Check sheet for the modelled part. Datum: model origin and axes. Units: mm. A direction names the side the tool comes from. Round coordinates to 2 decimals unless told otherwise and drop trailing zeros. Write each loop counter-clockwise with the first axis right and the second up, starting at its lowest first coordinate (ties: lowest second). Pieces come first, ordered by that corner, then holes. Notation, with made-up numbers: (-4, -32.5) -> (53, -32.5) arc R38 ccw to (53, 5.5) -> close; hole circle Ø7 at (-14, 20.25). An arc over 180 degrees is marked (long way). One line per item, written item: value.
from build123d import *

# Parameters (mm, degrees)
TORUS_R                = 1
CYLINDER_R             = 5.5
CYLINDER_DEPTH         = 36
FILLET_R               = 4
CYLINDER002_W          = 7
CYLINDER002_H          = 6
CYLINDER002_ANGLE      = 250
FILLET001_R            = 0.5
CUT001_PLACEMENT_ANGLE = 55
BOX_W                  = 8
BOX_H                  = 6
BOX_DEPTH              = 6
BOX001_W               = 2
BOX001_H               = 50
BOX001_DEPTH           = 10


with BuildPart() as toro:
    # Torus → Torus (revolve)
    with BuildSketch(Plane(origin=(0, 0, 26), x_dir=(1, 0, 0), z_dir=(0, -1, 0))):
        with Locations((6, 0)):
            Circle(TORUS_R)
    revolve(axis=Axis((0, 0, 26), (0, 0, 1)))


with BuildPart() as led:
    # Cylinder → Cylinder (new body)
    with BuildSketch(Plane.XY):
        Circle(CYLINDER_R)
    extrude(amount=CYLINDER_DEPTH)

    # Fillet
    fillet_edges = [led.edges().sort_by_distance(p)[0] for p in [
        (-5.5, 0, 36),
    ]]
    fillet(fillet_edges, radius=FILLET_R)

    # Cut: cut Toro
    add(toro.part, mode=Mode.SUBTRACT)


with BuildPart() as obj1:
    # Cylinder002 → Cylinder002 (revolve)
    with BuildSketch(Plane(origin=(0, 0, 4), x_dir=(1, 0, 0), z_dir=(0, -1, 0))):
        with Locations((3.5, 3)):
            Rectangle(CYLINDER002_W, CYLINDER002_H)
    revolve(axis=Axis((0, 0, 4), (0, 0, 1)), revolution_arc=CYLINDER002_ANGLE)

    # Fillet001
    fillet001_edges = [obj1.edges().sort_by_distance(p)[0] for p in [
        (-2.394141, -6.577848, 7),
        (7, 0, 7),
    ]]
    fillet(fillet001_edges, radius=FILLET001_R)


with BuildPart() as obj1_1:
    # Fillet001 placement: moved
    add(obj1.part.moved(Location((0, 0, 19))))

    # Cut001: cut led
    add(led.part, mode=Mode.SUBTRACT)


with BuildPart() as obj1_2:
    # Cut001 placement: moved
    add(obj1_1.part.moved(Location((0, 0, -26))).rotate(Axis((0, 0, -26), (0, 0, 1)), CUT001_PLACEMENT_ANGLE))


with BuildPart() as fusion:
    # Box → Box (new body)
    with BuildSketch(Plane(origin=(-14, -3, -3), x_dir=(1, 0, 0), z_dir=(0, 0, 1))):
        with Locations((4, 3)):
            Rectangle(BOX_W, BOX_H)
    extrude(amount=BOX_DEPTH)

    # Fusion: union obj1
    add(obj1_2.part)


with BuildPart() as obj2:
    # Box001 → Box001 (new body)
    with BuildSketch(Plane(origin=(-14, -25, -3), x_dir=(1, 0, 0), z_dir=(0, 0, 1))):
        with Locations((1, 25)):
            Rectangle(BOX001_W, BOX001_H)
    extrude(amount=BOX001_DEPTH)

    # Fusion001: union Fusion
    add(fusion.part)


solid = obj2.part
Item 1: Tool access check on faces 1 (the cylindrical face through (-5.497, 0.168, -1.948)), 2 (the flat face through (-6, 0, 3)), 3 (the flat face through (-9, -3, 0)), 4 (the flat face through (-9, 3, 0)). Record the directions out of +Z, -Z, +X, -X, +Y, -Y that give a thin tool (end or side, any length) a straight path to the whole face; none if there is none.
Answer:
face 1: -Z
face 2: +Z, +X, +Y, -Y
face 3: +Z, -Z, -Y
face 4: +Z, -Z, +Y
Item 2: Thickness scan on line 1 (Y direction, x = 0, z = 1.5); line 2 (X direction, y = 0, z = 2.1); line 3 (Z direction, x = -8.25, y = 0.5). Record the ranges inside material, lowest first.
Answer:
line 1: y = -7 to -5.5, 5.5 to 7
line 2: x = -14 to -5.5
line 3: z = -3 to 3
Item 3: Sectioned sample at C-C on y = 0. Enter the section's corners in (x, z).
Answer:
outline: (-14, -3) -> (-5.5, -3) -> (-5.5, -0.87) arc R1 ccw to (-5.5, 0.87) -> (-5.5, 3) -> (-12, 3) -> (-12, 7) -> (-14, 7) -> close
Item 4: Sectioned sample at A-A on x = 0. Enter the section's corners in (y, z), and give its area (3 significant figures).
Answer:
outline: (-7, -3) -> (-5.5, -3) -> (-5.5, -0.87) arc R1 ccw to (-5.5, 0.87) -> (-5.5, 3) -> (-7, 3) -> close; (5.5, -3) -> (7, -3) -> (7, 3) -> (5.5, 3) -> (5.5, 0.87) arc R1 ccw to (5.5, -0.87) -> close
area: 19.2 mm^2
Item 5: Sectioned sample at D-D on x = -10.25. Enter the section's corners in (y, z).
Answer:
outline: (-3, -3) -> (3, -3) -> (3, 3) -> (-3, 3) -> close
Item 6: Sectioned sample at B-B on z = 0. Enter the section's corners in (x, y), and give its area (3 significant figures).
Answer:
outline: (-14, -25) -> (-12, -25) -> (-12, -3) -> (-6.32, -3) arc R7 ccw to (3.56, -6.03) arc R0.5 ccw to (3.72, -5.31) -> (2.87, -4.1) arc R5 cw (long way) to (2.87, 4.1) -> (3.72, 5.31) arc R0.5 ccw to (3.56, 6.03) arc R7 ccw to (-6.32, 3) -> (-12, 3) -> (-12, 25) -> (-14, 25) -> close
area: 184 mm^2
Item 7: Mould release check, pull along X, two halves, no side actions. Record for faces 5 (the cylindrical face through (-2.13, -6.67, 0.04)), 6 (the flat face through (-13, 25, 2)), 7 (the flat face through (3.38, -4.83, 0.04)), 8 (the flat face through (-14, 0, 2)): pulls with the +X half, pulls with the -X half, needs draft (parallel to the pull), parting line crosses it, or undercut.
Answer:
face 5: undercut
face 6: needs draft
face 7: pulls with the +X half
face 8: pulls with the -X half
Item 8: Depth check by flat-ended pin: P1, Ø1.7, axis at x = -8.5, z = 1, coming from the -Y side; P2, Ø5, axis at y = -8, z = 4, coming from the +X side; P3, Ø5, axis at x = -4.5, z = 1, coming from the -Y side. Enter the tip coordinate at first touch or a pass-through.
Answer:
P1: stops at y = -3
P2: stops at x = 3.79
P3: stops at y = -6.71
